from build123d import *

# Parameters (mm, degrees)
F2_R     = 2.2225
F3_DEPTH = 25.4
F4_DEPTH = 35.56
F5_DEPTH = 38.1
F6_SIZE  = 3.175
F7_R     = 1.4986
F8_DEPTH = 8.001


with BuildPart() as f1:
    # F0 (on Front) → F1 (revolve)
    with BuildSketch(Plane.XZ):
        Polygon((0, 0), (14.9606, 0), (14.9606, 18.9992), (28.575, 18.9992), (28.575, 25.3492), (46.0375, 25.3492), (46.0375, 31.6992), (28.575, 31.6992), (28.575, 38.0492), (46.0375, 38.0492), (46.0375, 44.3992), (46.0375, 50.7492), (46.0375, 79.9592), (0, 79.9592), align=None)
    revolve(axis=Axis((0, 0, 39.9796), (0, 0, -1)))

    # F2 (on face) → F3 (cut)
    with BuildSketch(Plane.XY.offset(79.9592)):
        with BuildLine():
            Line((41.275, -9.525), (41.275, 9.525))
            ThreePointArc((41.275, 9.525), (31.75, 19.05), (22.225, 9.525))
            Line((22.225, 9.525), (22.225, -9.525))
            ThreePointArc((22.225, -9.525), (31.75, -19.05), (41.275, -9.525))
        make_face()
        with Locations((31.75, -9.525)):
            Circle(F2_R, mode=Mode.SUBTRACT)
        with Locations((31.75, 9.525)):
            Circle(F2_R, mode=Mode.SUBTRACT)
        with BuildLine():
            Line((-41.275, 9.525), (-41.275, -9.525))
            ThreePointArc((-41.275, -9.525), (-31.75, -19.05), (-22.225, -9.525))
            Line((-22.225, -9.525), (-22.225, 9.525))
            ThreePointArc((-22.225, 9.525), (-31.75, 19.05), (-41.275, 9.525))
        make_face()
        with Locations((-31.75, -9.525)):
            Circle(F2_R, mode=Mode.SUBTRACT)
        with Locations((-31.75, 9.525)):
            Circle(F2_R, mode=Mode.SUBTRACT)
    extrude(amount=-F3_DEPTH, mode=Mode.SUBTRACT)

    # F2 (on face) → F4 (cut)
    with BuildSketch(Plane.XY.offset(79.9592)):
        with BuildLine():
            Line((15.875, 9.1654355234), (15.875, -9.1654355234))
            ThreePointArc((15.875, -9.1654355234), (19.507052962, -23.9114029169), (29.5722317713, -35.2836295513))
            ThreePointArc((29.5722317713, -35.2836295513), (41.7185991281, -19.4681764179), (46.0375, 0))
            ThreePointArc((46.0375, 0), (41.7185991281, 19.4681764179), (29.5722317713, 35.2836295513))
            ThreePointArc((29.5722317713, 35.2836295513), (19.507052962, 23.9114029169), (15.875, 9.1654355234))
        make_face()
        with BuildLine():
            ThreePointArc((22.225, 9.525), (31.75, 19.05), (41.275, 9.525))
            Line((41.275, 9.525), (41.275, -9.525))
            ThreePointArc((41.275, -9.525), (31.75, -19.05), (22.225, -9.525))
            Line((22.225, -9.525), (22.225, 9.525))
        make_face(mode=Mode.SUBTRACT)
        with BuildLine():
            ThreePointArc((-15.875, 9.1654355234), (-19.507052962, 23.9114029169), (-29.5722317713, 35.2836295513))
            ThreePointArc((-29.5722317713, 35.2836295513), (-46.0375, 0), (-29.5722317713, -35.2836295513))
            ThreePointArc((-29.5722317713, -35.2836295513), (-19.507052962, -23.9114029169), (-15.875, -9.1654355234))
            Line((-15.875, -9.1654355234), (-15.875, 9.1654355234))
        make_face()
        with BuildLine():
            ThreePointArc((-22.225, -9.525), (-31.75, -19.05), (-41.275, -9.525))
            Line((-41.275, -9.525), (-41.275, 9.525))
            ThreePointArc((-41.275, 9.525), (-31.75, 19.05), (-22.225, 9.525))
            Line((-22.225, 9.525), (-22.225, -9.525))
        make_face(mode=Mode.SUBTRACT)
    extrude(amount=-F4_DEPTH, mode=Mode.SUBTRACT)

    # F2 (on face) → F5 (cut)
    with BuildSketch(Plane.XY.offset(79.9592)):
        with Locations((-31.75, 9.525)):
            Circle(F2_R)
        with Locations((-31.75, -9.525)):
            Circle(F2_R)
        with Locations((31.75, 9.525)):
            Circle(F2_R)
        with Locations((31.75, -9.525)):
            Circle(F2_R)
    extrude(amount=-F5_DEPTH, mode=Mode.SUBTRACT)

    # F6
    f6_edges = [f1.edges().sort_by_distance(p)[0] for p in [
        (0, -46.0375, 79.9592),
        (0, 46.0375, 79.9592),
    ]]
    chamfer(f6_edges, length=F6_SIZE)

    # F7 (on face) → F8 (cut)
    with BuildSketch(Plane(origin=(0, 0, 0), x_dir=(1, 0, 0), z_dir=(0, 0, -1))):
        with BuildLine():
            Line((4.0005, -4.0005), (4.0005, 4.0005))
            ThreePointArc((4.0005, 4.0005), (0, 8.001), (-4.0005, 4.0005))
            Line((-4.0005, 4.0005), (-4.0005, -4.0005))
            ThreePointArc((-4.0005, -4.0005), (0, -8.001), (4.0005, -4.0005))
        make_face()
        with Locations((-7.493, 0)):
            Circle(F7_R)
        with Locations((7.493, 0)):
            Circle(F7_R)
    extrude(amount=-F8_DEPTH, mode=Mode.SUBTRACT)


solid = f1.part
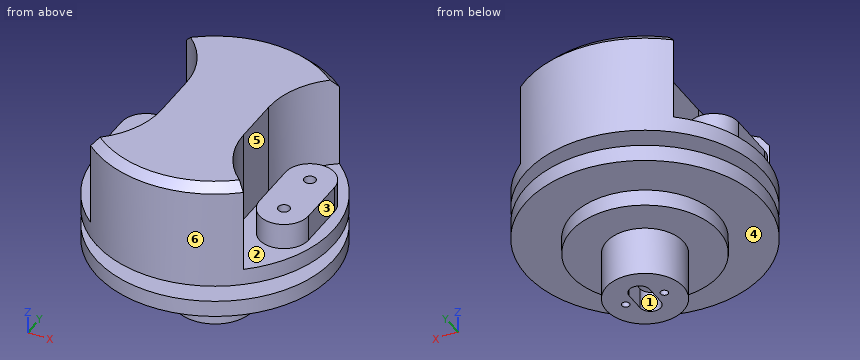
For this review, take the finished solid that the model builds, in its own axes (mm). Face numbers are marked on the shaded views. A direction names the side the tool comes from. Round coordinates to 2 decimals unless told otherwise and drop trailing zeros. Write each loop counter-clockwise with the first axis right and the second up, starting at its lowest first coordinate (ties: lowest second). Pieces come first, ordered by that corner, then holes. Notation, with made-up numbers: (44, 55.25) - (103, 55.25) arc R13 cw to (103, 73.25) - close; hole circle Ø8 at (66.5, -36). An arc over 180 degrees is marked (long way). Use a Markdown table: item, result.
Q1. Machinability: for the marked faces 1, 2 and 3, which of the approach directions +Z, -Z, +X, -X, +Y, -Y give a long, thin tool a straight path to every point of the face, cutting with its end or side? Answer none if there is none.
Derived:
| item | result |
|---|---|
| face 1 | -Z |
| face 2 | +Z |
| face 3 | +Z, +X, +Y, -Y |
Q2. We need section A-A (z = 48.5). State how many separate pieces and enclosed holes the cut face has, plus the area to 3 significant figures.
Derived:
| item | result |
|---|---|
| separate pieces | 3 |
| enclosed holes | 4 |
| area | 4,770 mm2 |
Q3. Wall thickness on line 1 along X through (y, z) = (0, 5); line 2 along Y through (x, z) = (-31.75, 51.25); line 3 along Z through (x, y) = (17.5, 24): over which ranges is each line inside the solid? List them lowest first.
Derived:
| item | result |
|---|---|
| line 1 | x = -14.96 to -8.99, -5.99 to -4, 4 to 5.99, 8.99 to 14.96 |
| line 2 | y = -19.05 to -11.75, -7.3 to 7.3, 11.75 to 19.05 |
| line 3 | z = 25.35 to 31.7, 38.05 to 79.96 |
Q4. We need section B-B (x = -31.75). Give the boundary of the cut face in (y, z), plus the area to 3 significant figures.
Derived:
| item | result |
|---|---|
| outline | (-33.34, 25.35) - (33.34, 25.35) - (33.34, 31.7) - (-33.34, 31.7) - close; (-33.34, 38.05) - (33.34, 38.05) - (33.34, 44.4) - (19.05, 44.4) - (19.05, 54.56) - (11.75, 54.56) - (11.75, 41.86) - (7.3, 41.86) - (7.3, 54.56) - (-7.3, 54.56) - (-7.3, 41.86) - (-11.75, 41.86) - (-11.75, 54.56) - (-19.05, 54.56) - (-19.05, 44.4) - (-33.34, 44.4) - close |
| area | 1,120 mm2 |
Q5. The part is to be moulded in two halves that separate along Y. For the marked faces 4, 5 and 6, say which applies: pulls with the +Y half, pulls with the -Y half, needs draft (parallel to the pull), parting line crosses it, or undercut.
Derived:
| item | result |
|---|---|
| face 4 | needs draft |
| face 5 | undercut |
| face 6 | parting line crosses it |
Q6. Clearance check with flat-ended pins moving along their axes: pin 1 (5 mm diameter, centred on x = -31.75, y = -9.525, fed in from +Z); pin 2 (10 mm diameter, centred on x = 12, z = 40, fed in from +Y); pin 3 (6.5 mm diameter, centred on y = -2, z = 4, fed in from +X). State where each tip first meets the part, or that it passes through.
Derived:
| item | result |
|---|---|
| pin 1 | stops at z = 54.56 |
| pin 2 | stops at y = 45.5 |
| pin 3 | stops at x = 14.96 |
Q7. We need section D-D (x = 0). Give the boundary of the cut face in (y, z) (1 decimal).
Derived:
| item | result |
|---|---|
| outline | (-46, 25.3) - (-28.6, 25.3) - (-28.6, 19) - (-15, 19) - (-15, 0) - (-8, 0) - (-8, 8) - (8, 8) - (8, 0) - (15, 0) - (15, 19) - (28.6, 19) - (28.6, 25.3) - (46, 25.3) - (46, 31.7) - (28.6, 31.7) - (28.6, 38) - (46, 38) - (46, 76.8) - (42.9, 80) - (-42.9, 80) - (-46, 76.8) - (-46, 38) - (-28.6, 38) - (-28.6, 31.7) - (-46, 31.7) - close |
Q8. We need section C-C (z = 5). Give the boundary of the cut face in (x, y).
Derived:
| item | result |
|---|---|
| outline | circle Ø29.92 at (0, 0); hole circle Ø3 at (-7.49, 0); hole (-4, -4) arc R4 ccw to (4, -4) - (4, 4) arc R4 ccw to (-4, 4) - close; hole circle Ø3 at (7.49, 0) |
